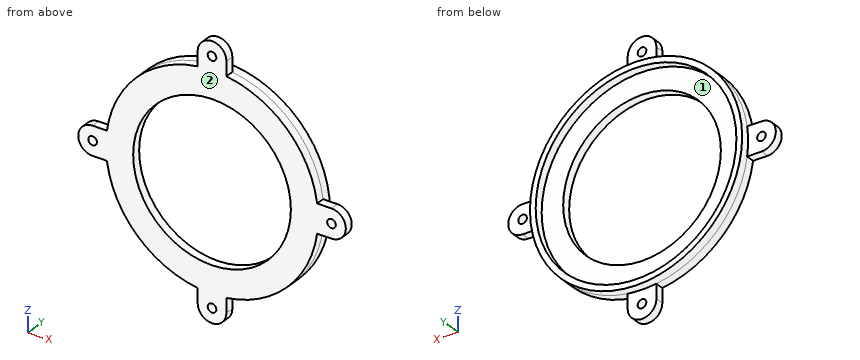
from build123d import *

# Parameters (mm, degrees)
SKETCH1_R           = 1.905
BOSS_EXTRUDE1_DEPTH = 3.81
SKETCH2_R           = 34.925
CUT_EXTRUDE2_DEPTH  = 4.81
SKETCH3_R           = 46.99
SKETCH3_R_2         = 44.45
BOSS_EXTRUDE2_DEPTH = 3.81


with BuildPart() as part:
    # Sketch1 → Boss-Extrude1 (new body)
    with BuildSketch(Plane(origin=(0, 0, 0), x_dir=(1, 0, 0), z_dir=(0, 1, 0))):
        with BuildLine():
            Line((46.558969061, 6.35), (52.908969061, 6.35))
            ThreePointArc((52.908969061, 6.35), (59.258969061, 0), (52.908969061, -6.35))
            Line((52.908969061, -6.35), (46.558969061, -6.35))
            ThreePointArc((46.558969061, -6.35), (33.226947648, -33.226947648), (6.35, -46.558969061))
            Line((6.35, -46.558969061), (6.35, -52.908969061))
            ThreePointArc((6.35, -52.908969061), (0, -59.258969061), (-6.35, -52.908969061))
            Line((-6.35, -52.908969061), (-6.35, -46.558969061))
            ThreePointArc((-6.35, -46.558969061), (-33.226947648, -33.226947648), (-46.558969061, -6.35))
            Line((-46.558969061, -6.35), (-52.908969061, -6.35))
            ThreePointArc((-52.908969061, -6.35), (-59.258969061, 0), (-52.908969061, 6.35))
            Line((-52.908969061, 6.35), (-46.558969061, 6.35))
            ThreePointArc((-46.558969061, 6.35), (-33.226947648, 33.226947648), (-6.35, 46.558969061))
            Line((-6.35, 46.558969061), (-6.35, 52.908969061))
            ThreePointArc((-6.35, 52.908969061), (0, 59.258969061), (6.35, 52.908969061))
            Line((6.35, 52.908969061), (6.35, 46.558969061))
            ThreePointArc((6.35, 46.558969061), (33.226947648, 33.226947648), (46.558969061, 6.35))
        make_face()
        with Locations((52.908969061, 0)):
            Circle(SKETCH1_R, mode=Mode.SUBTRACT)
        with Locations((0, -52.908969061)):
            Circle(SKETCH1_R, mode=Mode.SUBTRACT)
        with Locations((-52.908969061, 0)):
            Circle(SKETCH1_R, mode=Mode.SUBTRACT)
        with Locations((0, 52.908969061)):
            Circle(SKETCH1_R, mode=Mode.SUBTRACT)
    extrude(amount=BOSS_EXTRUDE1_DEPTH)

    # Sketch2 → Cut-Extrude2 (cut, through all)
    with BuildSketch(Plane(origin=(0, 3.81, 0), x_dir=(1, 0, 0), z_dir=(0, 1, 0))):
        Circle(SKETCH2_R)
    extrude(amount=-CUT_EXTRUDE2_DEPTH, mode=Mode.SUBTRACT)

    # Sketch3 → Boss-Extrude2 (add)
    with BuildSketch(Plane(origin=(0, 3.81, 0), x_dir=(1, 0, 0), z_dir=(0, 1, 0))):
        Circle(SKETCH3_R)
        Circle(SKETCH3_R_2, mode=Mode.SUBTRACT)
    extrude(amount=BOSS_EXTRUDE2_DEPTH)


solid = part.part
Input: part model. Units: mm. Frame: model coordinates. Face numbers are marked on the shaded views. Coordinates: 2 decimals unless noted, no trailing zeros. Order: outer loops, then holes, each group sorted by start corner. A loop starts at its lowest first (then second) coordinate and runs counter-clockwise, first axis right, second up. Notation, with made-up numbers: M -5,69.5 L 0,69.5 A24 cw 0,81.5 Z; hole C 83.5,40.25 d4. An arc over 180 degrees is marked long. Write item = value, one per line. Start each with the question number.
(1) Section A-A on x = 0. Output: boundary loops of the cut face in (y, z) (3 decimals).
(2) Line query: line 1 along X through (y, z) = (1.5, 0) (3 decimals); line 2 along Z through (x, y) = (0, 6.6). Output: solid intervals per line, ascending. Write a range as [from, to].
(3) Section D-D on x = 37. Output: boundary loops of the cut face in (y, z).
(4) Pull-direction query (X, two-part tool) for the marked faces 1 and 2; classes: released by +X, released by -X, zero draft, split by the parting line, or undercut.
(5) First-contact query: P1, Ø2, axis at x = -10.5, y = 3, coming from the +Z side; P2, Ø4, axis at y = 2.5, z = 50, coming from the -X side; P3, Ø1.5, axis at x = -5.5, y = 5.5, coming from the -Z side. Flat tips, straight axial feed; report the tip coordinate or a pass-through.
(6) Section B-B on y = 1.5. Output: boundary loops of the cut face in (x, z) (3 decimals).
(7) Section C-C on z = 0. Output: boundary loops of the cut face in (x, y) (3 decimals), and give its area (3 significant figures).
Result set:
q1.outline = M 0,-59.259 L 3.81,-59.259 L 3.81,-54.814 L 0,-54.814 Z; M 0,-51.004 L 3.81,-51.004 L 3.81,-46.99 L 7.62,-46.99 L 7.62,-44.45 L 3.81,-44.45 L 3.81,-34.925 L 0,-34.925 Z; M 0,34.925 L 3.81,34.925 L 3.81,44.45 L 7.62,44.45 L 7.62,46.99 L 3.81,46.99 L 3.81,51.004 L 0,51.004 Z; M 0,54.814 L 3.81,54.814 L 3.81,59.259 L 0,59.259 Z
q2.line_1 = [-59.259, -54.814], [-51.004, -34.925], [34.925, 51.004], [54.814, 59.259]
q2.line_2 = [-46.99, -44.45], [44.45, 46.99]
q3.outline = M 0,-28.97 L 7.62,-28.97 L 7.62,-24.63 L 3.81,-24.63 L 3.81,24.63 L 7.62,24.63 L 7.62,28.97 L 0,28.97 Z
q4.face_1 = undercut
q4.face_2 = zero draft
q5.P1 = 46.02
q5.P2 = -6.35
q5.P3 = -46.75
q6.outline = M -52.909,-6.35 L -46.559,-6.35 A46.99 ccw -6.35,-46.559 L -6.35,-52.909 A6.35 ccw 6.35,-52.909 L 6.35,-46.559 A46.99 ccw 46.559,-6.35 L 52.909,-6.35 A6.35 ccw 52.909,6.35 L 46.559,6.35 A46.99 ccw 6.35,46.559 L 6.35,52.909 A6.35 ccw -6.35,52.909 L -6.35,46.559 A46.99 ccw -46.559,6.35 L -52.909,6.35 A6.35 ccw Z; hole C -52.909,0 d3.81; hole C 0,0 d69.85; hole C 0,-52.909 d3.81; hole C 0,52.909 d3.81; hole C 52.909,0 d3.81
q7.outline = M -59.259,0 L -54.814,0 L -54.814,3.81 L -59.259,3.81 Z; M -51.004,0 L -34.925,0 L -34.925,3.81 L -44.45,3.81 L -44.45,7.62 L -46.99,7.62 L -46.99,3.81 L -51.004,3.81 Z; M 34.925,0 L 51.004,0 L 51.004,3.81 L 46.99,3.81 L 46.99,7.62 L 44.45,7.62 L 44.45,3.81 L 34.925,3.81 Z; M 54.814,0 L 59.259,0 L 59.259,3.81 L 54.814,3.81 Z
q7.area = 176 mm²
